Design review of the part built by this model. Coordinates are the model's own, in mm. Face numbers are marked on the shaded views. Round coordinates to 2 decimals unless told otherwise and drop trailing zeros. Order: outer loops, then holes, each group sorted by start corner. A loop starts at its lowest first (then second) coordinate and runs counter-clockwise, first axis right, second up. Notation, with made-up numbers: (40.5, 40) - (97.5, 40) arc R12 cw to (97.5, 50) - close; hole circle Ø3 at (89, 6.25). An arc over 180 degrees is marked (long way). Write item = value, one per line.
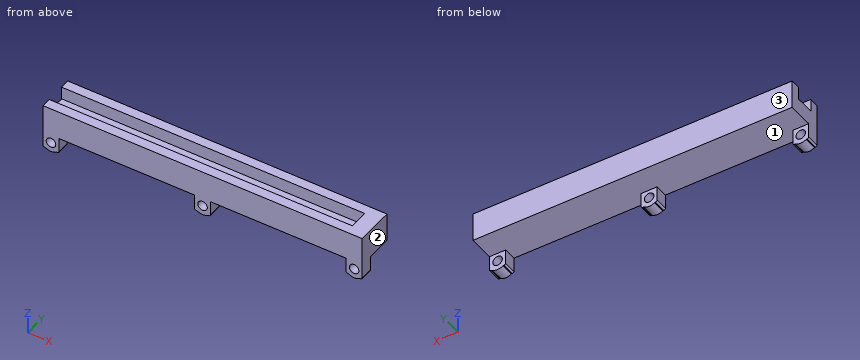
from build123d import *

# Parameters (mm, degrees)
ESQUISSE1_W        = 100
ESQUISSE1_H        = 12
BOSS_EXTRU_1_DEPTH = 5
BOSS_EXTRU_2_DEPTH = 4
ESQUISSE3_R        = 1.5
BOSS_EXTRU_3_DEPTH = 4


with BuildPart() as part:
    # Esquisse1 → Boss.-Extru.1 (new body)
    with BuildSketch(Plane.XY):
        Rectangle(ESQUISSE1_W, ESQUISSE1_H)
    extrude(amount=BOSS_EXTRU_1_DEPTH)

    # Esquisse2 → Boss.-Extru.2 (add)
    with BuildSketch(Plane.XY.offset(5)):
        Polygon((-50, 3), (45, 3), (45, -3), (-50, -3), (-50, -6), (50, -6), (50, 6), (-50, 6), align=None)
    extrude(amount=BOSS_EXTRU_2_DEPTH)

    # Esquisse3 → Boss.-Extru.3 (add)
    # profile 1 of 3: a face of its own
    with BuildSketch(Plane.XZ.offset(6)):
        with BuildLine():
            Line((-45.71168799, -5), (-45.5, -5))
            ThreePointArc((-45.5, -5), (-45.146446609, -4.853553391), (-45, -4.5))
            Line((-45, -4.5), (-45, 0))
            Line((-45, 0), (-50, 0))
            Line((-50, 0), (-50, -4.5))
            ThreePointArc((-50, -4.5), (-49.853553391, -4.853553391), (-49.5, -5))
            Line((-49.5, -5), (-49.28831201, -5))
            ThreePointArc((-49.28831201, -5), (-49.22893784, -5.008856171), (-49.174732569, -5.034653697))
            ThreePointArc((-49.174732569, -5.034653697), (-47.5, -5.545623601), (-45.825267431, -5.034653697))
            ThreePointArc((-45.825267431, -5.034653697), (-45.77106216, -5.008856171), (-45.71168799, -5))
        make_face()
        with Locations(Location((-47.5, -2.545623601, 0), (0, 0, 270))):
            Circle(ESQUISSE3_R, mode=Mode.SUBTRACT)
    # profile 2 of 3: a face of its own
    with BuildSketch(Plane.XZ.offset(6)):
        with BuildLine():
            Line((49.5, -5), (49.28831201, -5))
            ThreePointArc((49.28831201, -5), (49.22893784, -5.008856171), (49.174732569, -5.034653697))
            ThreePointArc((49.174732569, -5.034653697), (47.5, -5.545623601), (45.825267431, -5.034653697))
            ThreePointArc((45.825267431, -5.034653697), (45.77106216, -5.008856171), (45.71168799, -5))
            Line((45.71168799, -5), (45.5, -5))
            ThreePointArc((45.5, -5), (45.146446609, -4.853553391), (45, -4.5))
            Line((45, -4.5), (45, 0))
            Line((45, 0), (50, 0))
            Line((50, 0), (50, -4.5))
            ThreePointArc((50, -4.5), (49.853553391, -4.853553391), (49.5, -5))
        make_face()
        with Locations(Location((47.5, -2.545623601, 0), (0, 0, 90))):
            Circle(ESQUISSE3_R, mode=Mode.SUBTRACT)
    # profile 3 of 3: a face of its own
    with BuildSketch(Plane.XZ.offset(6)):
        with BuildLine():
            Line((-2.5, 0), (-2.5, -4.5))
            ThreePointArc((-2.5, -4.5), (-2.353553391, -4.853553391), (-2, -5))
            Line((-2, -5), (-1.78831201, -5))
            ThreePointArc((-1.78831201, -5), (-1.72893784, -5.008856171), (-1.674732569, -5.034653697))
            ThreePointArc((-1.674732569, -5.034653697), (0, -5.545623601), (1.674732569, -5.034653697))
            ThreePointArc((1.674732569, -5.034653697), (1.72893784, -5.008856171), (1.78831201, -5))
            Line((1.78831201, -5), (2, -5))
            ThreePointArc((2, -5), (2.353553391, -4.853553391), (2.5, -4.5))
            Line((2.5, -4.5), (2.5, 0))
            Line((2.5, 0), (-2.5, 0))
        make_face()
        with Locations(Location((0, -2.545623601, 0), (0, 0, 270))):
            Circle(ESQUISSE3_R, mode=Mode.SUBTRACT)
    extrude(amount=-BOSS_EXTRU_3_DEPTH)


solid = part.part
1) We need section B-B on y = -5. Give the number of separate pieces and of enclosed holes in the cut face, and give its area (3 significant figures).
Findings:
separate_pieces = 1
enclosed_holes = 3
area = 957 mm^2
2) To check wall thickness, follow L1, parallel to X at y = -3, z = -2.75; L2, parallel to Y at x = 6.5, z = 5.5; L3, parallel to Z at x = 47.5, y = -3.8. State the ranges of each line that lie inside material, in increasing order. Write a range as from..to.
Findings:
L1 = -50..-48.99, -46.01..-45, -2.5..-1.49, 1.49..2.5, 45..46.01, 48.99..50
L2 = -6..-3, 3..6
L3 = -5.55..-4.05, -1.05..9
3) We need section A-A on x = -47.5. Write out the cut boundary in (y, z), and give its area (3 significant figures).
Findings:
outline = (-6, -5.55) - (-2, -5.55) - (-2, -4.05) - (-6, -4.05) - close; (-6, -1.05) - (-2, -1.05) - (-2, 0) - (6, 0) - (6, 9) - (3, 9) - (3, 5) - (-3, 5) - (-3, 9) - (-6, 9) - close
area = 94.2 mm^2
4) The part is to be moulded in two halves that separate along X. For the marked faces 1, 2 and 3, say which applies: released by +X, released by -X, zero draft, split by the parting line, or undercut.
Findings:
face_1 = undercut
face_2 = released by +X
face_3 = zero draft
5) We need section C-C on z = 7. Write out the cut boundary in (x, y).
Findings:
outline = (-50, -6) - (50, -6) - (50, 6) - (-50, 6) - (-50, 3) - (45, 3) - (45, -3) - (-50, -3) - close
6) Clearance check with flat-ended pins moving along their axes: pin 1 Ø1.2 at (y, z) = (1, 7.5) entering from -X; pin 2 Ø2.5 at (x, z) = (-47.5, -2.55) entering from -Y; pin 3 Ø4 at (x, z) = (-47.5, -3.5) entering from +Y. State where each tip first meets the part, or that it passes through.
Findings:
pin_1 = 45
pin_2 = through
pin_3 = -2
7) We need section D-D on x = 47.5. Write out the cut boundary in (y, z), and give its area (3 significant figures).
Findings:
outline = (-6, -5.55) - (-2, -5.55) - (-2, -4.05) - (-6, -4.05) - close; (-6, -1.05) - (-2, -1.05) - (-2, 0) - (6, 0) - (6, 9) - (-6, 9) - close
area = 118 mm^2
